from build123d import *

# Parameters (mm, degrees)
F0_R     = 59
F0_R_2   = 55
F1_DEPTH = 7
F0_R_3   = 63
F0_R_4   = 20
F2_DEPTH = 5
F3_R     = 4.99999
F4_SIZE  = 1


# Not quite as in the source:
# - a fillet or chamfer is up to 0.001 mm smaller than in the source, because OpenCascade refuses the exact size


with BuildPart() as f1:
    # F0 (on Top) → F1 (new body)
    with BuildSketch(Plane.XY):
        Circle(F0_R)
        Circle(F0_R_2, mode=Mode.SUBTRACT)
    extrude(amount=F1_DEPTH)

    # F0 (on Top) → F2 (join)
    with BuildSketch(Plane.XY):
        Circle(F0_R_3)
        Circle(F0_R, mode=Mode.SUBTRACT)
        Circle(F0_R)
        Circle(F0_R_2, mode=Mode.SUBTRACT)
        Circle(F0_R_2)
        Circle(F0_R_4, mode=Mode.SUBTRACT)
    extrude(amount=-F2_DEPTH)

    # F3 (radius 5 in the source; OpenCascade refuses exactly that, so slightly less here)
    f3_edges = [f1.edges().sort_by_distance(p)[0] for p in [
        (-63, 0, -5),
    ]]
    fillet(f3_edges, radius=F3_R)

    # F4
    f4_edges = [f1.edges().sort_by_distance(p)[0] for p in [
        (-59, 0, 7),
    ]]
    chamfer(f4_edges, length=F4_SIZE)


solid = f1.part
Read the model definition and answer for the solid it produces. Units are mm, in the model's axes. A direction names the side the tool comes from. Coordinates: 2 decimals unless noted, no trailing zeros. Order: outer loops, then holes, each group sorted by start corner. A loop starts at its lowest first (then second) coordinate and runs counter-clockwise, first axis right, second up. Notation, with made-up numbers: (8.5, 27) -> (18.5, 27) arc R18 ccw to (18.5, 59) -> close; hole circle Ø8 at (81, -31.5). An arc over 180 degrees is marked (long way). Answer as a JSON object with one key per item and string values.
1) A cutting plane is placed at C-C, the plane z = 3.25. Determine the outline of the cut face in (x, y).
Model answer:
{"outline": "circle Ø118 at (0, 0); hole circle Ø110 at (0, 0)"}
2) Consider line 1 along Y through (x, z) = (0, 3.75); line 2 along Y through (x, z) = (44.5, 3.25); line 3 along Z through (x, y) = (-42, 16). Determine where each line is inside the solid, lowest interval first. Write a range as from..to.
Model answer:
{"line 1": "y = -59..-55, 55..59", "line 2": "y = -38.74..-32.32, 32.32..38.74", "line 3": "z = -5..0"}
3) The mould has two halves that part along Y. Classify faces 1 (the face through (-1, -25, -5)), 2 (the face through (56.275, 17.722, 2.958)), 3 (the face through (-11.923, -53.692, 3.451)): released by +Y, released by -Y, zero draft, split by the parting line, or undercut.
Model answer:
{"face 1": "zero draft", "face 2": "split by the parting line", "face 3": "undercut"}
4) A tool of negligible diameter and unlimited length cuts with its end or side. For faces 4 (the face through (-56.3, -18.4, 0)), 5 (the face through (51, -21, 7)), from which of +Z, -Z, +X, -X, +Y, -Y can it reach the whole face along a straight path? Write none if from no direction.
Model answer:
{"face 4": "+Z", "face 5": "+Z, +X, -X, +Y, -Y"}
5) Each of these flat-tipped pins is pushed along its axis until it touches: pin 1 (5 mm diameter, centred on x = -18, z = 4.5, fed in from +Y); pin 2 (5 mm diameter, centred on x = -32, z = -2, fed in from -Y); pin 3 (2 mm diameter, centred on x = -17.5, z = 3, fed in from +Y). Where does it stop, or does it pass through?
Model answer:
{"pin 1": "stops at y = 56.93", "pin 2": "stops at y = -55.44", "pin 3": "stops at y = 56.65"}
